Could you check a few things on this model? Use its own coordinates, in mm. A direction names the side the tool comes from. Coordinates: 2 decimals unless noted, no trailing zeros. Answer as a JSON object with one key per item and string values. Group by question number.
1) Please list where these lines run through material, in increasing order: line 1 along X through (y, z) = (18.75, 107); line 2 along X through (y, z) = (35, 28); line 3 along Y through (x, z) = (-18.25, 32.5).
2) Will these pins go through, and if not, where does the flat tip stop? pin 1 Ø4 at (y, z) = (28, 68.5) entering from -X; pin 2 Ø3 at (y, z) = (29.5, 68) entering from -X; pin 3 Ø6 at (y, z) = (28.5, 26.5) entering from -X.
3) We'd pull the mould along Y, two halves only. Please class faces 4 (the flat face through (-15.513, 20, 59)), 5 (the flat face through (-20.26, 23.11, 59)), 6 (the flat face through (-33, 37.302, 59)): released by +Y, released by -Y, zero draft, split by the parting line, or undercut.
4) On a 3-axis mill with a long thin cutter (end or side, diameter ignored), from which of +Z, -Z, +X, -X, +Y, -Y can I reach the whole of each face in a straight line? I mean faces 1 (the flat face through (-21.613, 26, 59)), 2 (the flat face through (-27, 23.402, 59)), 3 (the flat face through (-21, 19.102, 59)). Say none if no direction works.
```python
from build123d import *

# Parameters (mm, degrees)
V_SLOT_START                           = -5.085646751
V_SLOT_20X20X500_LINEAR_RAIL_OUTLINE_R = 2.1
V_SLOT_20X20X500_LINEAR_RAIL_DEPTH     = 500
SKETCH1_W                              = 20
SKETCH1_H                              = 370
CUT_EXTRUDE1_DEPTH                     = 497.589794047


# Read off the part's stored shape, not the designer's step: V-Slot 20x20x500 Linear Rail
with BuildPart() as part:
    # V-Slot 20x20x500 Linear Rail outline → V-Slot 20x20x500 Linear Rail (new body)
    with BuildSketch(Plane.XY.offset(V_SLOT_START)):
        with BuildLine():
            Line((-21.613469268, 24.462926439), (-21.613469268, 27.092266268))
            Line((-21.613469268, 27.092266268), (-21.823469268, 27.302266268))
            Line((-21.823469268, 27.302266268), (-21.613469268, 27.512266268))
            Line((-21.613469268, 27.512266268), (-21.613469268, 30.141606096))
            Line((-21.613469268, 30.141606096), (-18.952809096, 32.802266268))
            Line((-18.952809096, 32.802266268), (-17.313469268, 32.802266268))
            Line((-17.313469268, 32.802266268), (-17.313469268, 30.427266268))
            Line((-17.313469268, 30.427266268), (-16.968469268, 30.427266268))
            Line((-16.968469268, 30.427266268), (-15.513469268, 31.882266268))
            Line((-15.513469268, 31.882266268), (-15.513469268, 36.802266268))
            ThreePointArc((-15.513469268, 36.802266268), (-15.659915878, 37.155819658), (-16.013469268, 37.302266268))
            Line((-16.013469268, 37.302266268), (-20.933469268, 37.302266268))
            Line((-20.933469268, 37.302266268), (-22.388469268, 35.847266268))
            Line((-22.388469268, 35.847266268), (-22.388469268, 35.502266268))
            Line((-22.388469268, 35.502266268), (-20.013469268, 35.502266268))
            Line((-20.013469268, 35.502266268), (-20.013469268, 33.862926439))
            Line((-20.013469268, 33.862926439), (-22.67412944, 31.202266268))
            Line((-22.67412944, 31.202266268), (-25.303469268, 31.202266268))
            Line((-25.303469268, 31.202266268), (-25.513469268, 30.992266268))
            Line((-25.513469268, 30.992266268), (-25.723469268, 31.202266268))
            Line((-25.723469268, 31.202266268), (-28.352809096, 31.202266268))
            Line((-28.352809096, 31.202266268), (-31.013469268, 33.862926439))
            Line((-31.013469268, 33.862926439), (-31.013469268, 35.502266268))
            Line((-31.013469268, 35.502266268), (-28.638469268, 35.502266268))
            Line((-28.638469268, 35.502266268), (-28.638469268, 35.847266268))
            Line((-28.638469268, 35.847266268), (-30.093469268, 37.302266268))
            Line((-30.093469268, 37.302266268), (-35.013469268, 37.302266268))
            ThreePointArc((-35.013469268, 37.302266268), (-35.367022659, 37.155819658), (-35.513469268, 36.802266268))
            Line((-35.513469268, 36.802266268), (-35.513469268, 31.882266268))
            Line((-35.513469268, 31.882266268), (-34.058469268, 30.427266268))
            Line((-34.058469268, 30.427266268), (-33.713469268, 30.427266268))
            Line((-33.713469268, 30.427266268), (-33.713469268, 32.802266268))
            Line((-33.713469268, 32.802266268), (-32.07412944, 32.802266268))
            Line((-32.07412944, 32.802266268), (-29.413469268, 30.141606096))
            Line((-29.413469268, 30.141606096), (-29.413469268, 27.512266268))
            Line((-29.413469268, 27.512266268), (-29.203469268, 27.302266268))
            Line((-29.203469268, 27.302266268), (-29.413469268, 27.092266268))
            Line((-29.413469268, 27.092266268), (-29.413469268, 24.462926439))
            Line((-29.413469268, 24.462926439), (-32.07412944, 21.802266268))
            Line((-32.07412944, 21.802266268), (-33.713469268, 21.802266268))
            Line((-33.713469268, 21.802266268), (-33.713469268, 24.177266268))
            Line((-33.713469268, 24.177266268), (-34.058469268, 24.177266268))
            Line((-34.058469268, 24.177266268), (-35.513469268, 22.722266268))
            Line((-35.513469268, 22.722266268), (-35.513469268, 17.802266268))
            ThreePointArc((-35.513469268, 17.802266268), (-35.367022659, 17.448712877), (-35.013469268, 17.302266268))
            Line((-35.013469268, 17.302266268), (-30.093469268, 17.302266268))
            Line((-30.093469268, 17.302266268), (-28.638469268, 18.757266268))
            Line((-28.638469268, 18.757266268), (-28.638469268, 19.102266268))
            Line((-28.638469268, 19.102266268), (-31.013469268, 19.102266268))
            Line((-31.013469268, 19.102266268), (-31.013469268, 20.741606096))
            Line((-31.013469268, 20.741606096), (-28.352809096, 23.402266268))
            Line((-28.352809096, 23.402266268), (-25.723469268, 23.402266268))
            Line((-25.723469268, 23.402266268), (-25.513469268, 23.612266268))
            Line((-25.513469268, 23.612266268), (-25.303469268, 23.402266268))
            Line((-25.303469268, 23.402266268), (-22.67412944, 23.402266268))
            Line((-22.67412944, 23.402266268), (-20.013469268, 20.741606096))
            Line((-20.013469268, 20.741606096), (-20.013469268, 19.102266268))
            Line((-20.013469268, 19.102266268), (-22.388469268, 19.102266268))
            Line((-22.388469268, 19.102266268), (-22.388469268, 18.757266268))
            Line((-22.388469268, 18.757266268), (-20.933469268, 17.302266268))
            Line((-20.933469268, 17.302266268), (-16.013469268, 17.302266268))
            ThreePointArc((-16.013469268, 17.302266268), (-15.659915877, 17.448712878), (-15.513469268, 17.802266268))
            Line((-15.513469268, 17.802266268), (-15.513469268, 22.722266268))
            Line((-15.513469268, 22.722266268), (-16.968469268, 24.177266268))
            Line((-16.968469268, 24.177266268), (-17.313469268, 24.177266268))
            Line((-17.313469268, 24.177266268), (-17.313469268, 21.802266268))
            Line((-17.313469268, 21.802266268), (-18.952809096, 21.802266268))
            Line((-18.952809096, 21.802266268), (-21.613469268, 24.462926439))
        make_face()
        with Locations((-25.513469268, 27.302266268)):
            Circle(V_SLOT_20X20X500_LINEAR_RAIL_OUTLINE_R, mode=Mode.SUBTRACT)
    extrude(amount=V_SLOT_20X20X500_LINEAR_RAIL_DEPTH)

    # Sketch1 → Cut-Extrude1 (cut, through all)
    with BuildSketch(Plane(origin=(0, 37.302266268, 0), x_dir=(1, 0, 0), z_dir=(0, 1, 0))):
        with Locations((-25.513469268, -309.914353249)):
            Rectangle(SKETCH1_W, SKETCH1_H)
    extrude(amount=-CUT_EXTRUDE1_DEPTH, mode=Mode.SUBTRACT)


solid = part.part
```
Here are the results:
{
 "1": {"line 1": "x = -35.51 to -28.65, -22.38 to -15.51", "line 2": "x = -35.51 to -31.01, -20.01 to -15.51", "line 3": "y = 17.3 to 21.8, 32.8 to 37.3"},
 "2": {"pin 1": "stops at x = -29.41", "pin 2": "stops at x = -34.63", "pin 3": "stops at x = -35.13"},
 "3": {"face 4": "zero draft", "face 5": "undercut", "face 6": "released by +Y"},
 "4": {"face 1": "+Z, -Z, +X", "face 2": "+Z, -Z, -Y", "face 3": "+Z, -Z"}
}
